Autodesk Inventor part; units mm, degrees
ref_plane "YZ Plane" through (0, 0, 0) normal (1, 0, 0) x (0, 1, 0)
ref_plane "XZ Plane" through (0, 0, 0) normal (0, 1, 0) x (-1, 0, 0)
ref_plane "XY Plane" through (0, 0, 0) normal (0, 0, 1) x (1, 0, 0)
sketch "Boceto1" plane through (0, 0, 0) normal (0, 0, 1) x (1, 0, 0)
  line L0 (9, 9) -> (-9, 9)
  line L1 (-9, 9) -> (-9, -9)
  line L2 (-9, -9) -> (9, -9)
  line L3 (9, -9) -> (9, 9)
  line L4 (9, 9) -> (-9, -9) construction
  line L5 (-9, 9) -> (9, -9) construction
  point P0 (0, 0)
  dimension "d0" = 18
extrude "Extrusión1" add sketch "Boceto1" along normal blind 18
fillet "Empalme1" radius 2 12 edges at (9, 0, 0) (9, 9, 9) (9, 0, 18) (9, -9, 9) (0, -9, 0) (0, -9, 18) (-9, -9, 9) (-9, 0, 0) (-9, 0, 18) (-9, 9, 9) (0, 9, 0) (0, 9, 18)
sketch "Boceto2" plane through (0, 0, 0) normal (0, 0, -1) x (-1, 0, 0)
  circle A0 centre (0, 0) radius 4.025
  dimension "d4" = 8.05
extrude "Extrusión2" cut sketch "Boceto2" against normal blind 5
sketch "Boceto3" plane through (-7, -9, 2) normal (0, -1, 0) x (1, 0, 0)
  circle A0 centre (7, 7) radius 4.025
  line L0 (14, 0) -> (0, 0)
  line L1 (0, 0) -> (0, 14)
  point P0 (7, -2)
  dimension "d7" = 8.05
  dimension "d8" = 7
  dimension "d9" = 7
extrude "Extrusión3" cut sketch "Boceto3" against normal blind 5
properties part number "Hombro"
Geometry: final body of the model. Coordinates: model frame, mm. A direction names the side the tool comes from. Coordinates: 2 decimals unless noted, no trailing zeros. Order: outer loops, then holes, each group sorted by start corner. A loop starts at its lowest first (then second) coordinate and runs counter-clockwise, first axis right, second up. Notation, with made-up numbers: (6, 10.25) -> (42, 10.25) arc R36 ccw to (42, 48.25) -> close; hole circle Ø1 at (-17.75, 43). An arc over 180 degrees is marked (long way). Answer in a Markdown table with one row per item.
Item 1: Section B-B on y = -5. Output: boundary loops of the cut face in (x, z) (3 decimals).
Return value:
| item | result |
|---|---|
| outline | (-9, 2) arc R2 ccw to (-7, 0) -> (7, 0) arc R2 ccw to (9, 2) -> (9, 16) arc R2 ccw to (7, 18) -> (-7, 18) arc R2 ccw to (-9, 16) -> close; hole circle Ø8.05 at (0, 9) |
Item 2: Draft query along X for faces 1 (the flat face through (-9, 0, 9)), 2 (the flat face through (0, 0, 5)), 3 (the flat face through (-3, -3, 0)), 4 (the flat face through (9, 0, 9)). Return one class per face: released by +X, released by -X, zero draft, split by the parting line, or undercut.
Return value:
| item | result |
|---|---|
| face 1 | released by -X |
| face 2 | undercut |
| face 3 | zero draft |
| face 4 | released by +X |
Item 3: Access query for faces 5 (the cylindrical face through (-0.1, 8.4, 17.43)), 6 (the cylindrical face through (-0.87, -6.54, 5.07)). Directions: +Z, -Z, +X, -X, +Y, -Y. A direction counts if a zero-diameter tool reaches every point of the face in a straight line with its end or side. Return the directions, or none.
Return value:
| item | result |
|---|---|
| face 5 | +Z, +X, -X, +Y |
| face 6 | -Y |
Item 4: Section C-C on z = 9. Output: boundary loops of the cut face in (x, y) (3 decimals), plus the area to 3 significant figures.
Return value:
| item | result |
|---|---|
| outline | (-9, -7) arc R2 ccw to (-7, -9) -> (-4.025, -9) -> (-4.025, -4) -> (4.025, -4) -> (4.025, -9) -> (7, -9) arc R2 ccw to (9, -7) -> (9, 7) arc R2 ccw to (7, 9) -> (-7, 9) arc R2 ccw to (-9, 7) -> close |
| area | 280 mm² |
Item 5: Ray query, L1, parallel to X at y = 0, z = 2.8 (3 decimals); L2, parallel to Z at x = 0, y = -6 (3 decimals); L3, parallel to Y at x = -3.25, z = 7.5. Return the intervals inside material, ascending.
Return value:
| item | result |
|---|---|
| L1 | x = -9 to -4.025, 4.025 to 9 |
| L2 | z = 0 to 4.975, 13.025 to 18 |
| L3 | y = -4 to 9 |
Item 6: Section A-A on x = 0. Output: boundary loops of the cut face in (y, z) (3 decimals).
Return value:
| item | result |
|---|---|
| outline | (-9, 2) arc R2 ccw to (-7, 0) -> (-4.025, 0) -> (-4.025, 4.975) -> (-9, 4.975) -> close; (-9, 13.025) -> (-4, 13.025) -> (-4, 5) -> (4.025, 5) -> (4.025, 0) -> (7, 0) arc R2 ccw to (9, 2) -> (9, 16) arc R2 ccw to (7, 18) -> (-7, 18) arc R2 ccw to (-9, 16) -> close |
Item 7: Section D-D on y = 0. Output: boundary loops of the cut face in (x, z) (3 decimals).
Return value:
| item | result |
|---|---|
| outline | (-9, 2) arc R2 ccw to (-7, 0) -> (-4.025, 0) -> (-4.025, 5) -> (4.025, 5) -> (4.025, 0) -> (7, 0) arc R2 ccw to (9, 2) -> (9, 16) arc R2 ccw to (7, 18) -> (-7, 18) arc R2 ccw to (-9, 16) -> close |
Item 8: Contact query for a flat-ended pin moving along its axis: P1, Ø2.5, axis at x = 0, y = 1, coming from the -Z side. Output: stop coordinate, or through.
Return value:
| item | result |
|---|---|
| P1 | stops at z = 5 |
